Work out the finished part from the listing and answer in its coordinate system (mm). A direction names the side the tool comes from. Round coordinates to 2 decimals unless told otherwise and drop trailing zeros. Loops run counter-clockwise (first coordinate to the right, second up) from the corner with the lowest first, then second, coordinate; pieces in that order, holes last. Notation, with made-up numbers: M -20,-7.5 L 37,-7.5 A28 cw 37,23.5 Z; hole C 78,2.25 d7. An arc over 180 degrees is marked long. One line per item, written item: value.
```python
from build123d import *

# Parameters (mm, degrees)
SKETCH1_W            = 90
SKETCH1_H            = 90
BOSS_EXTRUDE1_DEPTH  = 25.4
SKETCH2_R            = 5.08
CUT_EXTRUDE1_DEPTH   = 50.8
LPATTERN1_COUNT      = 2
LPATTERN1_PITCH      = 64.516
LPATTERN1_COUNT_DIR2 = 2
LPATTERN1_PITCH_DIR2 = 64.516
SKETCH4_R            = 4.445
CUT_EXTRUDE3_DEPTH   = 26.4
SKETCH5_R            = 8.89
CUT_EXTRUDE4_DEPTH   = 7.62


with BuildPart() as part:
    # Sketch1 → Boss-Extrude1 (new body)
    with BuildSketch(Plane(origin=(0, 0, 0), x_dir=(1, 0, 0), z_dir=(0, 1, 0))):
        Rectangle(SKETCH1_W, SKETCH1_H)
    extrude(amount=BOSS_EXTRUDE1_DEPTH)

    # Sketch2 → Cut-Extrude1 (cut)
    with BuildSketch(Plane(origin=(0, 25.4, 0), x_dir=(-1, 0, 0), z_dir=(0, 1, 0))):
        with Locations((32.3, -32.3)):
            Circle(SKETCH2_R)
    cut_extrude1 = extrude(amount=-CUT_EXTRUDE1_DEPTH, mode=Mode.SUBTRACT)

    # LPattern1: Cut-Extrude1 2 × 2
    with Locations(*[(i * LPATTERN1_PITCH, 0, j * LPATTERN1_PITCH_DIR2) for i in range(LPATTERN1_COUNT) for j in range(LPATTERN1_COUNT_DIR2) if (i, j) != (0, 0)]):
        add(cut_extrude1, mode=Mode.SUBTRACT)

    # Sketch4 → Cut-Extrude3 (cut, through all)
    with BuildSketch(Plane(origin=(0, 25.4, 0), x_dir=(1, 0, 0), z_dir=(0, 1, 0))):
        with Locations((0, 20.574)):
            Circle(SKETCH4_R)
        with Locations((0, -20.574)):
            Circle(SKETCH4_R)
    extrude(amount=-CUT_EXTRUDE3_DEPTH, mode=Mode.SUBTRACT)

    # Sketch5 → Cut-Extrude4 (cut)
    with BuildSketch(Plane.XZ):
        with Locations((0, -20.574)):
            Circle(SKETCH5_R)
        with Locations((0, 20.574)):
            Circle(SKETCH5_R)
    extrude(amount=-CUT_EXTRUDE4_DEPTH, mode=Mode.SUBTRACT)


solid = part.part
```
1) Find section C-C (y = 23.5). Give the vertices of the cut face in (x, z) (3 decimals), then the cut area to 3 significant figures.
Check values:
outline: M -45,-45 L 45,-45 L 45,45 L -45,45 Z; hole C -32.3,-32.3 d10.16; hole C -32.3,32.216 d10.16; hole C 0,-20.574 d8.89; hole C 0,20.574 d8.89; hole C 32.216,-32.3 d10.16; hole C 32.216,32.216 d10.16
area: 7,650 mm2
2) Find section B-B (z = -32.3). Give the vertices of the cut face in (x, y), then the cut area to 3 significant figures.
Check values:
outline: M -45,0 L -37.38,0 L -37.38,25.4 L -45,25.4 Z; M -27.22,0 L 27.14,0 L 27.14,25.4 L -27.22,25.4 Z; M 37.3,0 L 45,0 L 45,25.4 L 37.3,25.4 Z
area: 1,770 mm2
3) Find the intervals of material crossed by probe 1 along Z at (x, y) = (0, 6.25); probe 2 along Z at (x, y) = (0, 21); probe 3 along X at (y, z) = (23, 32.5), in increasing order. Write a range as from..to.
Check values:
probe 1: -45..-29.46, -11.68..11.68, 29.46..45
probe 2: -45..-25.02, -16.13..16.13, 25.02..45
probe 3: -45..-37.37, -27.23..27.14, 37.29..45
4) Find section D-D (x = -32.3). Give the vertices of the cut face in (y, z).
Check values:
outline: M 0,-45 L 25.4,-45 L 25.4,-37.38 L 0,-37.38 Z; M 0,-27.22 L 25.4,-27.22 L 25.4,27.14 L 0,27.14 Z; M 0,37.3 L 25.4,37.3 L 25.4,45 L 0,45 Z
5) Find section A-A (x = 0). Give the vertices of the cut face in (y, z), then the cut area to 3 significant figures.
Check values:
outline: M 0,-45 L 25.4,-45 L 25.4,-25.02 L 7.62,-25.02 L 7.62,-29.46 L 0,-29.46 Z; M 0,-11.68 L 7.62,-11.68 L 7.62,-16.13 L 25.4,-16.13 L 25.4,16.13 L 7.62,16.13 L 7.62,11.68 L 0,11.68 Z; M 0,29.46 L 7.62,29.46 L 7.62,25.02 L 25.4,25.02 L 25.4,45 L 0,45 Z
area: 1,700 mm2
6) Each of these flat-tipped pins is pushed along its axis until it touches: pin 1 (6 mm diameter, centred on x = 32.216, z = 32.216, fed in from +Y); pin 2 (11.5 mm diameter, centred on x = 0, z = -20.574, fed in from -Y). Where does it stop, or does it pass through?
Check values:
pin 1: through
pin 2: y = 7.62
7) For faces 1 (the face through (-1, 25.4, -1)), 2 (the face through (-1.16, 3.76, -11.76)), determine the directions among +Z, -Z, +X, -X, +Y, -Y from which every point of the face is accessible in a straight line to the end or side of a thin tool.
Check values:
face 1: +Z, -Z, +X, -X, +Y
face 2: -Y
8) The mould has two halves that part along Z. Classify faces 3 (the face through (-1, 13, 45)), 4 (the face through (-0.579, 16.634, 16.167)), 5 (the face through (-45, 13, 1)): +Z half, -Z half, draft (parallel to the pull), parting line (faces both ways), or undercut.
Check values:
face 3: +Z half
face 4: undercut
face 5: draft
